```python
from build123d import *

# Parameters (mm, degrees)
F1_DEPTH = 2133.6


with BuildPart() as f1:
    # F0 (on Front) → F1 (new body)
    with BuildSketch(Plane.XZ):
        with BuildLine():
            ThreePointArc((-0.27041, 226.486726), (-115.087389, -68.746585), (-389.148504, -227.605492))
            Line((-389.148504, -227.605492), (387.464732, -228.379771))
            ThreePointArc((387.464732, -228.379771), (141.321633, -61.134424), (58.43205, 224.674512))
            ThreePointArc((58.43205, 224.674512), (59.008561, 243.586212), (40.115219, 242.573104))
            Line((40.115219, 242.573104), (15.73921, 242.573104))
            ThreePointArc((15.73921, 242.573104), (-0.17472, 242.401296), (-0.27041, 226.486726))
        make_face()
    extrude(amount=F1_DEPTH)


solid = f1.part
```
Can you work these out from the model? Positions are in its coordinate system, mm. Give positions to 0.01 mm unless a question says otherwise; leave off trailing zeros. Loops run counter-clockwise (first coordinate to the right, second up) from the corner with the lowest first, then second, coordinate; pieces in that order, holes last. Notation, with made-up numbers: M -18.5,-0.5 L 31.5,-0.5 A16 cw 31.5,27.5 Z; hole C 48.5,70.5 d2. An arc over 180 degrees is marked long. Answer in a Markdown table with one row per item.
1. Suppose I cut it at B-B on z = -95. Write out the boundary of the cut face in (x, y), plus the area to 3 significant figures.
Taken from the geometry:
| item | result |
|---|---|
| outline | M -139.33,-2133.6 L 168.58,-2133.6 L 168.58,0 L -139.33,0 Z |
| area | 657,000 mm² |
2. Suppose I cut it at A-A on x = -141. Write out the boundary of the cut face in (y, z), plus the area to 3 significant figures.
Taken from the geometry:
| item | result |
|---|---|
| outline | M -2133.6,-227.85 L 0,-227.85 L 0,-96.67 L -2133.6,-96.67 Z |
| area | 280,000 mm² |
3. If I drill on line 1 along X through (y, z) = (-192.5, 169); line 2 along Z through (x, y) = (139, -1386.5); line 3 along Z through (x, y) = (-150, -1265.5), over which ranges is the centre line in solid material (lowest first)?
Taken from the geometry:
| item | result |
|---|---|
| line 1 | x = -5.69 to 58.43 |
| line 2 | z = -228.13 to -57.91 |
| line 3 | z = -227.84 to -105.4 |
4. Suppose I cut it at C-C on y = -695.5. Write out the boundary of the cut face in (x, z).
Taken from the geometry:
| item | result |
|---|---|
| outline | M -389.15,-227.61 L 387.46,-228.38 A438.91 cw 58.43,224.67 A12.85 ccw long 40.12,242.57 L 15.74,242.57 A11.35 ccw -0.27,226.49 A478.61 cw Z |
5. For pin 1 Ø3 at (y, z) = (-801.5, -15) entering from +X; pin 2 Ø3 at (y, z) = (-385, 73.5) entering from +X; pin 3 Ø4 at (x, y) = (-305, -401) entering from -Z, each with a flat end and sliding along its axis, tell me the tip position at first contact or that it passes through.
Taken from the geometry:
| item | result |
|---|---|
| pin 1 | stops at x = 112.85 |
| pin 2 | stops at x = 75.66 |
| pin 3 | stops at z = -227.69 |
